Here's how the part is built. I have some questions about the finished solid (model axes, mm). Give positions to 0.01 mm unless a question says otherwise; leave off trailing zeros. Order: outer loops, then holes, each group sorted by start corner. A loop starts at its lowest first (then second) coordinate and runs counter-clockwise, first axis right, second up. Notation, with made-up numbers: M -25.75,-37 L 16.25,-37 A12 cw 16.25,-26 Z; hole C -23,-27 d9. An arc over 180 degrees is marked long. One line per item, written item: value. Start each with the question number.
from build123d import *

# Parameters (mm, degrees)
ESBO_O1_R                = 4.765
RESSALTO_EXTRUS_O1_DEPTH = 8
FILETE1_R                = 1


with BuildPart() as part:
    # Esboço1 → Ressalto-extrusão1 (new body)
    with BuildSketch(Plane.XY):
        Polygon((8, 0), (4, 6.92820323), (-4, 6.92820323), (-8, 0), (-4, -6.92820323), (4, -6.92820323), align=None)
        Circle(ESBO_O1_R, mode=Mode.SUBTRACT)
    extrude(amount=RESSALTO_EXTRUS_O1_DEPTH)

    # Filete1
    filete1_edges = [part.edges().sort_by_distance(p)[0] for p in [
        (0, 6.92820323, 8),
        (4, -6.92820323, 4),
        (-4, -6.92820323, 4),
        (-8, 0, 4),
        (-4, 6.92820323, 4),
        (4, 6.92820323, 4),
        (8, 0, 4),
        (-6, 3.464101615, 8),
        (-6, -3.464101615, 8),
        (-4.765, 0, 0),
        (-4.765, 0, 8),
        (0, -6.92820323, 8),
        (6, -3.464101615, 8),
        (0, -6.92820323, 0),
        (-6, -3.464101615, 0),
        (-6, 3.464101615, 0),
        (6, 3.464101615, 8),
        (0, 6.92820323, 0),
        (6, 3.464101615, 0),
        (6, -3.464101615, 0),
    ]]
    fillet(filete1_edges, radius=FILETE1_R)


solid = part.part
Item 1: Will these pins go through, and if not, where does the flat tip stop? P1, Ø3, axis at x = -4.5, y = -2, coming from the -Z side; P2, Ø2, axis at x = 1.5, y = 1, coming from the -Z side.
Item 2: I want a section at A-A on x = 0. Write out the boundary of the cut face in (y, z) (3 decimals).
Item 3: I want a section at C-C on z = 7.5. Write out the boundary of the cut face in (x, y), plus the area to 3 significant figures.
Item 4: I want a section at B-B on z = 5.75. Write out the boundary of the cut face in (x, y) (3 decimals).
Item 5: We'd pull the mould along X, two halves only. Please class faces 1 (the face through (-0.62, 4.724, 3.958)), 2 (the face through (-5.976, 3.506, 3.958)), 3 (the face through (5.976, -3.506, 3.958)): +X half, -X half, draft (parallel to the pull), parting line (faces both ways), or undercut.
Item 6: Please list where these lines run through material, in increasing order: probe 1 along Y at (x, z) = (0, 3.2) (3 decimals); probe 2 along Y at (x, z) = (4.25, 1.25); probe 3 along X at (y, z) = (4.25, 1). Write a range as [from, to].
Answer below:
1. P1: stops at z = 0
1. P2: passes through
2. outline: M -6.928,1 A1 ccw -5.928,0 L -5.765,0 A1 ccw -4.765,1 L -4.765,7 A1 ccw -5.765,8 L -5.928,8 A1 ccw -6.928,7 Z; M 4.765,1 A1 ccw 5.765,0 L 5.928,0 A1 ccw 6.928,1 L 6.928,7 A1 ccw 5.928,8 L 5.765,8 A1 ccw 4.765,7 Z
3. outline: M -7.6,-0.43 L -4.17,-6.36 A0.87 ccw -3.42,-6.79 L 3.42,-6.79 A0.87 ccw 4.17,-6.36 L 7.6,-0.43 A0.87 ccw 7.6,0.43 L 4.17,6.36 A0.87 ccw 3.42,6.79 L -3.42,6.79 A0.87 ccw -4.17,6.36 L -7.6,0.43 A0.87 ccw Z; hole C 0,0 d9.8
3. area: 84.3 mm²
4. outline: M -7.711,-0.5 L -4.289,-6.428 A1 ccw -3.423,-6.928 L 3.423,-6.928 A1 ccw 4.289,-6.428 L 7.711,-0.5 A1 ccw 7.711,0.5 L 4.289,6.428 A1 ccw 3.423,6.928 L -3.423,6.928 A1 ccw -4.289,6.428 L -7.711,0.5 A1 ccw Z; hole C 0,0 d9.53
5. face 1: undercut
5. face 2: -X half
5. face 3: +X half
6. probe 1: y = [-6.928, -4.765], [4.765, 6.928]
6. probe 2: y = [-6.49, -2.15], [2.15, 6.49]
6. probe 3: x = [-5.55, -2.15], [2.15, 5.55]
